Part model, mm, in its own coordinate system. Coordinates: 2 decimals unless noted, no trailing zeros. Order: outer loops, then holes, each group sorted by start corner. A loop starts at its lowest first (then second) coordinate and runs counter-clockwise, first axis right, second up. Notation, with made-up numbers: M 74,-24 L 126,-24 A18 cw 126,-8 Z; hole C 12,5.5 d8. An arc over 180 degrees is marked long. Answer in a Markdown table with one row per item. Add a question column.
from build123d import *

# Parameters (mm, degrees)
SKETCH1_R           = 1.575
BOSS_EXTRUDE1_DEPTH = 3
L_EK1_SCALE         = 2


with BuildPart() as part:
    # Sketch1 → Boss-Extrude1 (new body)
    with BuildSketch(Plane(origin=(0, 0, 0), x_dir=(1, 0, 0), z_dir=(0, 1, 0))):
        with BuildLine():
            Line((0, -5), (23.998875872, -5))
            ThreePointArc((23.998875872, -5), (24.467345461, -4.883479623), (24.826642543, -4.561072489))
            Line((24.826642543, -4.561072489), (28.564941326, 0.954149161))
            ThreePointArc((28.564941326, 0.954149161), (28.766036178, 1.172359953), (29.022312673, 1.321950886))
            Line((29.022312673, 1.321950886), (40.929553216, 6.070049343))
            ThreePointArc((40.929553216, 6.070049343), (41.304486381, 6.141164834), (41.678758689, 6.066649533))
            Line((41.678758689, 6.066649533), (47.144586244, 3.829406729))
            Line((47.144586244, 3.829406729), (48.06174016, 3.086958957))
            Line((48.06174016, 3.086958957), (48.804187932, 4.004112872))
            Line((48.804187932, 4.004112872), (49.721341848, 3.2616651))
            Line((49.721341848, 3.2616651), (50.46378962, 4.178819016))
            Line((50.46378962, 4.178819016), (51.380943536, 3.436371244))
            Line((51.380943536, 3.436371244), (52.123391308, 4.35352516))
            Line((52.123391308, 4.35352516), (53.040545224, 3.611077387))
            Line((53.040545224, 3.611077387), (53.782992996, 4.528231303))
            Line((53.782992996, 4.528231303), (54.700146912, 3.785783531))
            Line((54.700146912, 3.785783531), (55.442594685, 4.702937447))
            Line((55.442594685, 4.702937447), (52.341745918, 12.244834503))
            ThreePointArc((52.341745918, 12.244834503), (52.137055639, 12.558350103), (51.831402108, 12.774604725))
            Line((51.831402108, 12.774604725), (46.024183924, 15.419882568))
            ThreePointArc((46.024183924, 15.419882568), (45.628323444, 15.509674561), (45.229386093, 15.434727162))
            Line((45.229386093, 15.434727162), (20.032711481, 5.075121772))
            ThreePointArc((20.032711481, 5.075121772), (19.846254378, 5.018960187), (19.652448068, 5))
            Line((19.652448068, 5), (0, 5))
            ThreePointArc((0, 5), (-5, 0), (0, -5))
        make_face()
        with Locations(Location((0, 0, 0), (0, 0, 270))):
            Circle(SKETCH1_R, mode=Mode.SUBTRACT)
        with Locations(Location((22, 0, 0), (0, 0, 270))):
            Circle(SKETCH1_R, mode=Mode.SUBTRACT)
    extrude(amount=BOSS_EXTRUDE1_DEPTH)


with BuildPart() as part_1:
    # Ölçek1: scaled about (24.645515764, 1.5, -3.692559234)
    add(part.part.scale(L_EK1_SCALE).moved(Location((-24.645515764, -1.5, 3.692559234))))


solid = part_1.part
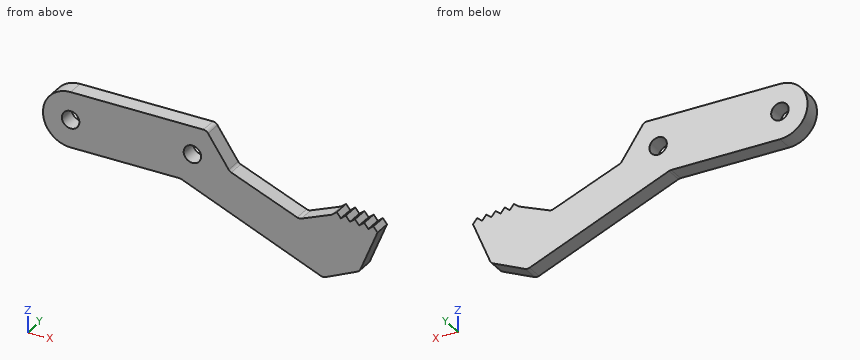
(1) Wall check: line 1 (X direction, y = 1.8, z = 4); line 2 (X direction, y = 2.5, z = 6.5); line 3 (Z direction, x = 13.5, y = -0.95). Give the ranges that are in metal, low to high.
(2) Slice it at C-C (z = -1). List the corners of the cut face in (x, y).
(3) Drop flat-ended pins along their axis: P1, Ø2, axis at y = 0, z = 6.5, coming from the +X side; P2, Ø1.8, axis at x = -6, y = 2, coming from the -Z side. Give the stop position or say it passes through.
(4) Slice it at B-B (x = -12.5). List the corners of the cut face in (y, z).
(5) Slice it at A-A (y = 3.6). List the corners of the cut face in (x, z).
Computed:
| question | item | result |
|---|---|---|
| 1 | line 1 | x = -34.64 to -27.78, -21.51 to 16.22, 22.49 to 30.98 |
| 1 | line 2 | x = -34.24 to -26.07, -23.22 to 17.93, 20.78 to 29.29 |
| 1 | line 3 | z = -6.31 to 13.69 |
| 2 | outline | M -33.48,-1.5 L 38.54,-1.5 L 38.54,4.5 L -33.48,4.5 Z |
| 3 | P1 | stops at x = 29.97 |
| 3 | P2 | stops at z = -6.31 |
| 4 | outline | M -1.5,-6.31 L 4.5,-6.31 L 4.5,13.69 L -1.5,13.69 Z |
| 5 | outline | M -24.65,-6.31 L 14.66,-6.31 A2 cw 15.42,-6.46 L 65.81,-27.18 A2 ccw 67.4,-27.15 L 79.02,-21.86 A2 ccw 80.04,-20.8 L 86.24,-5.71 L 84.75,-3.88 L 82.92,-5.36 L 81.44,-3.53 L 79.6,-5.01 L 78.12,-3.18 L 76.28,-4.67 L 74.8,-2.83 L 72.96,-4.32 L 71.48,-2.48 L 69.64,-3.97 L 58.71,-8.44 A2 cw 57.21,-8.45 L 33.4,1.05 A2 cw 32.48,1.78 L 25.01,12.81 A2 ccw 23.35,13.69 L -24.65,13.69 A10 ccw Z; hole C -24.65,3.69 d6.3; hole C 19.35,3.69 d6.3 |
